```python
from build123d import *

# Parameters (mm, degrees)
SKETCH_1_W          = 340
SKETCH_1_H          = 255
EXTRUDE_1_DEPTH     = 3
EXTRUDE_2_DEPTH     = 2
SKETCH_3_R          = 21.75
SKETCH_3_W          = 50
SKETCH_3_H          = 17
CUT_EXTRUDE_1_DEPTH = 5
EXTRUDE_START       = -3
SKETCH_4_W          = 340
SKETCH_4_H          = 20
EXTRUDE_3_DEPTH     = 3
FILLET_1_R          = 3


with BuildPart() as part:
    # 草圖1 → 填料-伸長1 (new body)
    with BuildSketch(Plane(origin=(0, 0, 0), x_dir=(1, 0, 0), z_dir=(0, 1, 0))):
        Rectangle(SKETCH_1_W, SKETCH_1_H)
    extrude(amount=EXTRUDE_1_DEPTH)

    # 草圖2 → 填料-伸長2 (add)
    with BuildSketch(Plane.XZ):
        Polygon((-166.5, 100.5), (-143, 124), (143, 124), (166.5, 100.5), (166.5, -124), (-166.5, -124), align=None)
    extrude(amount=EXTRUDE_2_DEPTH)

    # 草圖3 → 除料-伸長1 (cut)
    with BuildSketch(Plane(origin=(0, 3, 0), x_dir=(1, 0, 0), z_dir=(0, 1, 0))):
        with Locations(Location((-127.5, 85, 0), (0, 0, 270))):
            Circle(SKETCH_3_R)
        with Locations(Location((-42.5, 85, 0), (0, 0, 270))):
            Circle(SKETCH_3_R)
        with Locations(Location((-127.5, 0, 0), (0, 0, 270))):
            Circle(SKETCH_3_R)
        with Locations(Location((-42.5, 0, 0), (0, 0, 270))):
            Circle(SKETCH_3_R)
        with Locations(Location((-127.5, -85, 0), (0, 0, 270))):
            Circle(SKETCH_3_R)
        with Locations(Location((-42.5, -85, 0), (0, 0, 270))):
            Circle(SKETCH_3_R)
        with Locations(Location((127.5, -85, 0), (0, 0, 90))):
            Circle(SKETCH_3_R)
        with Locations(Location((42.5, -85, 0), (0, 0, 90))):
            Circle(SKETCH_3_R)
        with Locations(Location((42.5, 0, 0), (0, 0, 90))):
            Circle(SKETCH_3_R)
        with Locations(Location((127.5, 0, 0), (0, 0, 90))):
            Circle(SKETCH_3_R)
        with Locations(Location((127.5, 85, 0), (0, 0, 90))):
            Circle(SKETCH_3_R)
        with Locations(Location((42.5, 85, 0), (0, 0, 90))):
            Circle(SKETCH_3_R)
        with Locations((0, 119)):
            Rectangle(SKETCH_3_W, SKETCH_3_H)
    extrude(amount=-CUT_EXTRUDE_1_DEPTH, mode=Mode.SUBTRACT)

    # 草圖4 → 填料-伸長3 (add)
    with BuildSketch(Plane(origin=(0, 3, 0), x_dir=(1, 0, 0), z_dir=(0, 1, 0)).offset(EXTRUDE_START)):
        with Locations((0, -137.5)):
            Rectangle(SKETCH_4_W, SKETCH_4_H)
    extrude(amount=EXTRUDE_3_DEPTH)

    # 圓角1
    fillet_1_edges = [part.edges().sort_by_distance(p)[0] for p in [
        (-170, 1.5, 147.5),
        (170, 1.5, 147.5),
        (-25, 1.5, -127.5),
        (-25, 0.5, -110.5),
        (25, 1.5, -127.5),
        (25, 0.5, -110.5),
        (-170, 1.5, -127.5),
        (170, 1.5, -127.5),
    ]]
    fillet(fillet_1_edges, radius=FILLET_1_R)


solid = part.part
```
Geometry check sheet. Reference: the model listing, model coordinates, mm. A direction names the side the tool comes from. Give positions to 0.01 mm unless a question says otherwise; leave off trailing zeros. Write each loop counter-clockwise with the first axis right and the second up, starting at its lowest first coordinate (ties: lowest second). Pieces come first, ordered by that corner, then holes. Notation, with made-up numbers: (45.5, 48) -> (91.5, 48) arc R20 ccw to (91.5, 57) -> close; hole circle Ø10 at (81.5, 84.5). An arc over 180 degrees is marked (long way). One line per question, with ' | ' between items.
Item 1: Scan lines: line 1 along X through (y, z) = (0.6, -85); line 2 along Z through (x, y) = (127.5, 0.55); line 3 along X through (y, z) = (-0.5, 85). Record each from-to range of solid material in increasing order.
Determined:
line 1: -170 to -149.25, -105.75 to -64.25, -20.75 to 20.75, 64.25 to 105.75, 149.25 to 170 | line 2: -127.5 to -106.75, -63.25 to -21.75, 21.75 to 63.25, 106.75 to 147.5 | line 3: -166.5 to -149.25, -105.75 to -64.25, -20.75 to 20.75, 64.25 to 105.75, 149.25 to 166.5
Item 2: Sectioned sample at B-B, the plane x = -127.5. Record the boundary of the cut face in (y, z).
Determined:
outline: (-2, -124) -> (0, -124) -> (0, -127.5) -> (3, -127.5) -> (3, -106.75) -> (-2, -106.75) -> close; (-2, -63.25) -> (3, -63.25) -> (3, -21.75) -> (-2, -21.75) -> close; (-2, 21.75) -> (3, 21.75) -> (3, 63.25) -> (-2, 63.25) -> close; (-2, 106.75) -> (3, 106.75) -> (3, 147.5) -> (0, 147.5) -> (0, 124) -> (-2, 124) -> close
Item 3: Access from +Z, -Z, +X, -X, +Y, -Y to the whole of each face (thin tool, end or side, straight path). Record for faces 1 (the flat face through (155, -1, 112)), 2 (the cylindrical face through (35.967, 0.535, -105.746)).
Determined:
face 1: +Z, +X, -Y | face 2: +Y, -Y
Item 4: Sectioned sample at A-A, the plane z = 0. Record the boundary of the cut face in (x, y), plus the area to 3 significant figures.
Determined:
outline: (-170, 0) -> (-166.5, 0) -> (-166.5, -2) -> (-149.25, -2) -> (-149.25, 3) -> (-170, 3) -> close; (-105.75, -2) -> (-64.25, -2) -> (-64.25, 3) -> (-105.75, 3) -> close; (-20.75, -2) -> (20.75, -2) -> (20.75, 3) -> (-20.75, 3) -> close; (64.25, -2) -> (105.75, -2) -> (105.75, 3) -> (64.25, 3) -> close; (149.25, -2) -> (166.5, -2) -> (166.5, 0) -> (170, 0) -> (170, 3) -> (149.25, 3) -> close | area: 816 mm^2
Item 5: Draft check along Z on faces 3 (the flat face through (-1, 0, 132)), 4 (the flat face through (-155, -1, 112)), 5 (the cylindrical face through (-109.16, 0.54, 11.69)). Enter one of: released by +Z, released by -Z, zero draft, split by the parting line, or undercut.
Determined:
face 3: zero draft | face 4: released by +Z | face 5: undercut
Item 6: Sectioned sample at D-D, the plane x = 74. Record the boundary of the cut face in (y, z).
Determined:
outline: (-2, -124) -> (0, -124) -> (0, -127.5) -> (3, -127.5) -> (3, 147.5) -> (0, 147.5) -> (0, 124) -> (-2, 124) -> close
Item 7: Sectioned sample at C-C, the plane y = -1.2. State how many separate pieces and enclosed holes the cut face has, plus the area to 3 significant figures.
Determined:
separate pieces: 1 | enclosed holes: 12 | area: 63,500 mm^2
Item 8: Depth check by flat-ended pin: pin 1 (1.5 mm diameter, centred on x = 0.5, y = -0.5, fed in from -Z); pin 2 (1 mm diameter, centred on x = -75.5, y = -1, fed in from +Z); pin 3 (0.6 mm diameter, centred on x = 83, y = -1.5, fed in from -Z). Enter the tip coordinate at first touch or a pass-through.
Determined:
pin 1: z = -110.5 | pin 2: z = 124 | pin 3: z = -124
